Check sheet for the drawn part. Datum: minimum x, y, z corner. Units: mm. A direction names the side the tool comes from. Give positions to 0.01 mm unless a question says otherwise; leave off trailing zeros. Order: outer loops, then holes, each group sorted by start corner. A loop starts at its lowest first (then second) coordinate and runs counter-clockwise, first axis right, second up. Notation, with made-up numbers: (21.25, -18.75) -> (49.25, -18.75) arc R18 ccw to (49.25, -2.75) -> close; hole circle Ø1 at (-35, -18). An arc over 180 degrees is marked (long way). Answer in a Markdown table with one row per item. Add a question column.
(1) Cross-section at C-C (x = 12.5). Record the cut outline in (y, z), then the cut area to 3 significant figures.
(2) Set-up check for the marked faces 1, 2, 3, 4 and 5: record each of +Z, -Z, +X, -X, +Y, -Y from which the full face is reachable in a straight line by a thin tool's end or side.
(3) Release check for a two-part mould opening along Y. For the marked faces 6, 7 and 8 record: released by +Y, released by -Y, zero draft, split by the parting line, or undercut.
(4) Cross-section at B-B (y = 23). Record the cut outline in (x, z), then the cut area to 3 significant figures.
(5) Cross-section at D-D (x = 27). Record the cut outline in (y, z).
(6) Cross-section at A-A (y = 15). Record the cut outline in (x, z).
(7) Go/stop test with flat-tipped pins: pin 1 (5 mm diameter, centred on y = 14.5, z = 15, fed in from +X); pin 2 (5 mm diameter, centred on y = 25.5, z = 6, fed in from -X); pin 3 (1.2 mm diameter, centred on x = 21, y = 14.5, fed in from -Z); pin 4 (3 mm diameter, centred on y = 4, z = 16.6, fed in from +X). Record where each tip stops, or that it passes through.
(8) Thickness scan on L1, parallel to Y at x = 20.9, z = 16.6; L2, parallel to X at y = 5.5, z = 21.5; L3, parallel to Z at x = 11, y = 15. Record the ranges inside material, lowest first. Write a range as [from, to].
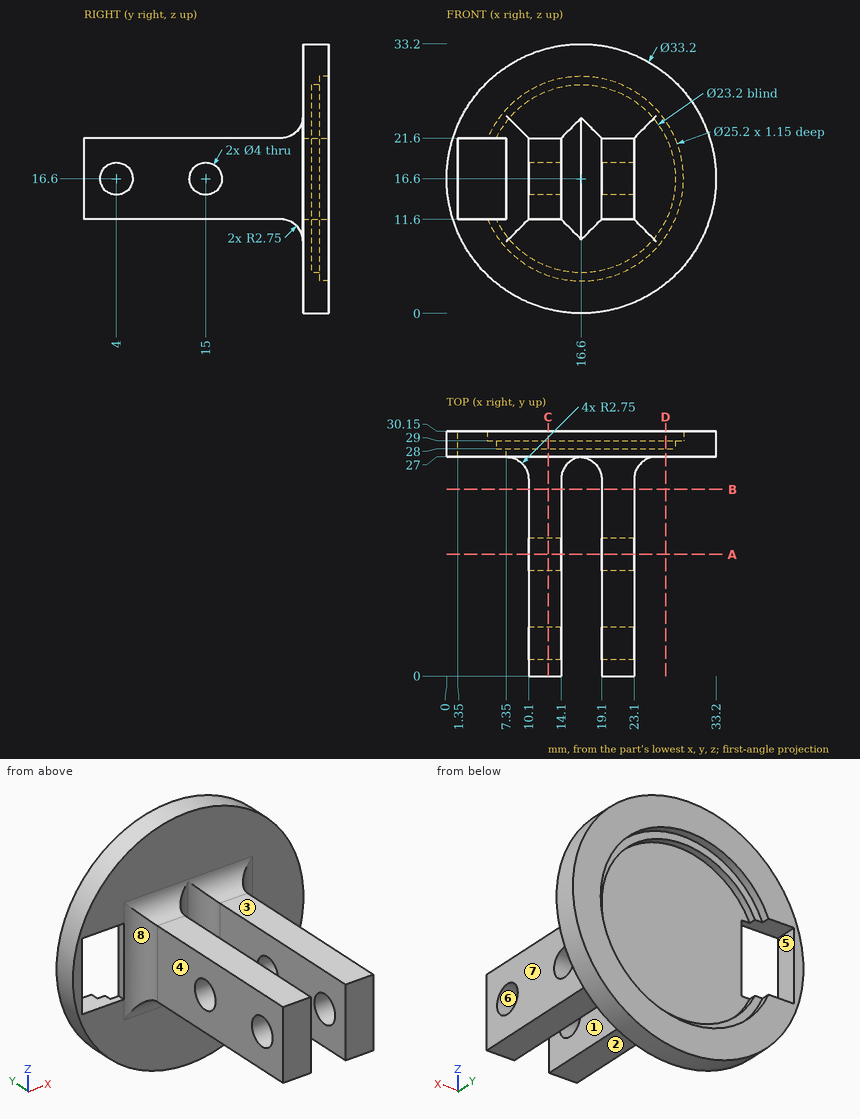
Answer below:
| question | item | result |
|---|---|---|
| 1 | outline | (0, 11.6) -> (24.25, 11.6) arc R2.75 cw to (27, 8.85) -> (27, 0.51) -> (30.15, 0.51) -> (30.15, 4.69) -> (29, 4.69) -> (29, 5.75) -> (28, 5.75) -> (28, 27.45) -> (29, 27.45) -> (29, 28.51) -> (30.15, 28.51) -> (30.15, 32.69) -> (27, 32.69) -> (27, 24.35) arc R2.75 cw to (24.25, 21.6) -> (0, 21.6) -> close; hole circle Ø4 at (4, 16.6); hole circle Ø4 at (15, 16.6) |
| 1 | area | 300 mm² |
| 2 | face 1 | +Z, -Z, -Y |
| 2 | face 2 | -Z, +X, -X, -Y |
| 2 | face 3 | +Z, +X, -X, -Y |
| 2 | face 4 | +Z, -Z, -X, -Y |
| 2 | face 5 | +Y, -Y |
| 3 | face 6 | undercut |
| 3 | face 7 | zero draft |
| 3 | face 8 | released by -Y |
| 4 | outline | (10.1, 11.6) -> (14.1, 11.6) -> (14.1, 21.6) -> (10.1, 21.6) -> close; (19.1, 11.6) -> (23.1, 11.6) -> (23.1, 21.6) -> (19.1, 21.6) -> close |
| 4 | area | 80.0 mm² |
| 5 | outline | (27, 3.66) -> (30.15, 3.66) -> (30.15, 9.49) -> (29, 9.49) -> (29, 11.46) -> (28, 11.46) -> (28, 21.74) -> (29, 21.74) -> (29, 23.71) -> (30.15, 23.71) -> (30.15, 29.54) -> (27, 29.54) -> close |
| 6 | outline | (10.1, 11.6) -> (14.1, 11.6) -> (14.1, 14.6) -> (10.1, 14.6) -> close; (10.1, 18.6) -> (14.1, 18.6) -> (14.1, 21.6) -> (10.1, 21.6) -> close; (19.1, 11.6) -> (23.1, 11.6) -> (23.1, 14.6) -> (19.1, 14.6) -> close; (19.1, 18.6) -> (23.1, 18.6) -> (23.1, 21.6) -> (19.1, 21.6) -> close |
| 7 | pin 1 | stops at x = 23.1 |
| 7 | pin 2 | stops at x = 2.4 |
| 7 | pin 3 | stops at z = 11.6 |
| 7 | pin 4 | passes through |
| 8 | L1 | y = [0, 2], [6, 13], [17, 28] |
| 8 | L2 | x = [10.1, 14.1], [19.1, 23.1] |
| 8 | L3 | z = [11.6, 14.6], [18.6, 21.6] |
